Here's the drawing with two shaded views (mm, measured from the low corner). I have some questions. Round coordinates to 2 decimals unless told otherwise and drop trailing zeros. Order: outer loops, then holes, each group sorted by start corner. A loop starts at its lowest first (then second) coordinate and runs counter-clockwise, first axis right, second up. Notation, with made-up numbers: (56.5, 45.5) -> (84.5, 45.5) arc R22 cw to (84.5, 82.5) -> close; hole circle Ø6 at (58, 33). An arc over 180 degrees is marked (long way). One line per question, with ' | ' between items.
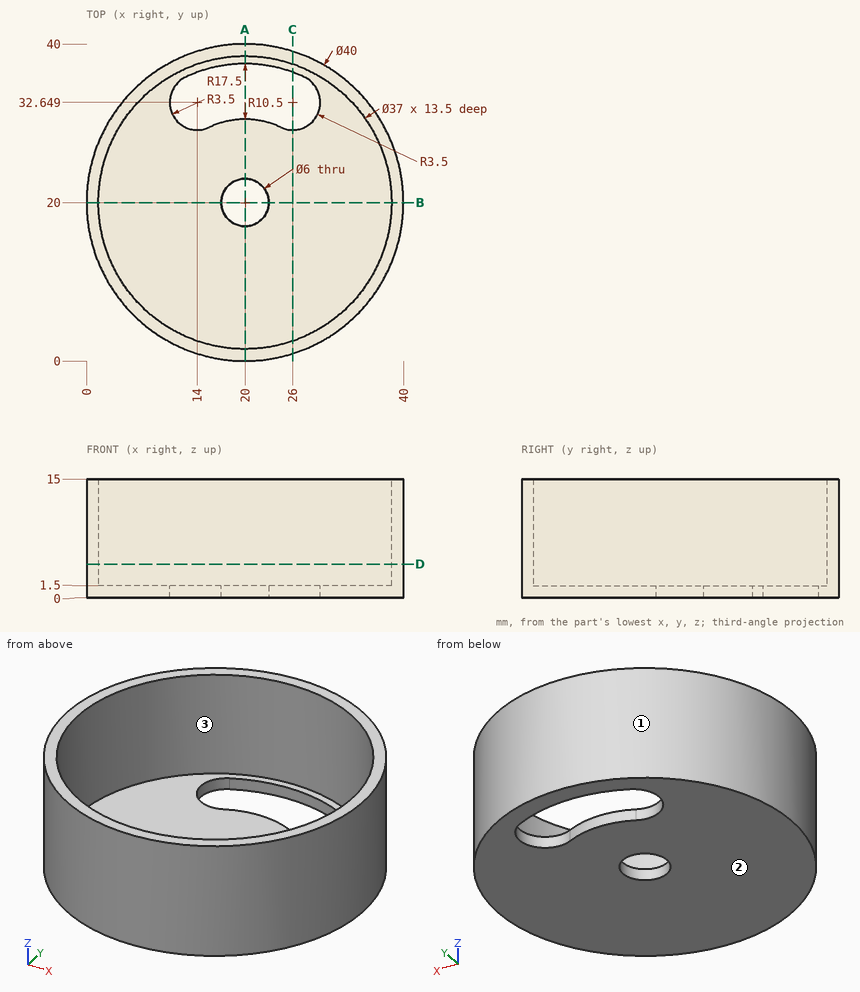
1. I'm going to push flat-ended pins straight in: pin 1 (2 mm diameter, centred on x = 29, z = 13, fed in from +Y); pin 2 (5 mm diameter, centred on x = 25.5, z = 11.5, fed in from +Y); pin 3 (1 mm diameter, centred on y = 28, z = 8.5, fed in from +X); pin 4 (10 mm diameter, centred on x = 22, y = 35.5, fed in from -Z). Where does each tip first touch, or does it pass through?
From the geometry:
pin 1: stops at y = 38.33 | pin 2: stops at y = 39.77 | pin 3: stops at x = 38.54 | pin 4: stops at z = 0
2. I want a section at A-A on x = 20. List the corners of the cut face in (y, z) for me, and give its area (3 significant figures).
From the geometry:
outline: (0, 0) -> (17, 0) -> (17, 1.5) -> (1.5, 1.5) -> (1.5, 15) -> (0, 15) -> close; (23, 0) -> (30.5, 0) -> (30.5, 1.5) -> (23, 1.5) -> close; (37.5, 0) -> (40, 0) -> (40, 15) -> (38.5, 15) -> (38.5, 1.5) -> (37.5, 1.5) -> close | area: 81.0 mm²
3. I want a section at B-B on y = 20. List the corners of the cut face in (x, z) for me, and give its area (3 significant figures).
From the geometry:
outline: (0, 0) -> (17, 0) -> (17, 1.5) -> (1.5, 1.5) -> (1.5, 15) -> (0, 15) -> close; (23, 0) -> (40, 0) -> (40, 15) -> (38.5, 15) -> (38.5, 1.5) -> (23, 1.5) -> close | area: 91.5 mm²
4. If we mould it in two halves opening along Y, with no side actions, what happens to the marked faces 1, 2 and 3? For each: pulls with the +Y half, pulls with the -Y half, needs draft (parallel to the pull), parting line crosses it, or undercut.
From the geometry:
face 1: parting line crosses it | face 2: needs draft | face 3: undercut
5. I want a section at D-D on z = 4.25. List the corners of the cut face in (x, y) for me.
From the geometry:
outline: circle Ø40 at (20, 20); hole circle Ø37 at (20, 20)
6. I need wall thicknesses on probe 1 along Z at (x, y) = (29, 28.5); probe 2 along X at (y, z) = (30, 11.5); probe 3 along X at (y, z) = (24, 4.25). Which ranges of each line are inside material? Lowest first, please.
From the geometry:
probe 1: z = 0 to 1.5 | probe 2: x = 2.68 to 4.44, 35.56 to 37.32 | probe 3: x = 0.4 to 1.94, 38.06 to 39.6
7. I want a section at C-C on x = 26. List the corners of the cut face in (y, z) for me.
From the geometry:
outline: (0.92, 0) -> (29.15, 0) -> (29.15, 1.5) -> (2.5, 1.5) -> (2.5, 15) -> (0.92, 15) -> close; (36.44, 0) -> (39.08, 0) -> (39.08, 15) -> (37.5, 15) -> (37.5, 1.5) -> (36.44, 1.5) -> close
